Can you work these out from the drawing? Everything is in mm from the part's minimum corner. A direction names the side the tool comes from. Round coordinates to 2 decimals unless told otherwise and drop trailing zeros. Loops run counter-clockwise (first coordinate to the right, second up) from the corner with the lowest first, then second, coordinate; pieces in that order, holes last. Notation, with made-up numbers: M 63,2.5 L 95,2.5 A7 cw 95,14.5 Z; hole C -33,71.5 d10. An arc over 180 degrees is marked long. One line per question, with ' | ' between items. Start each with the question number.
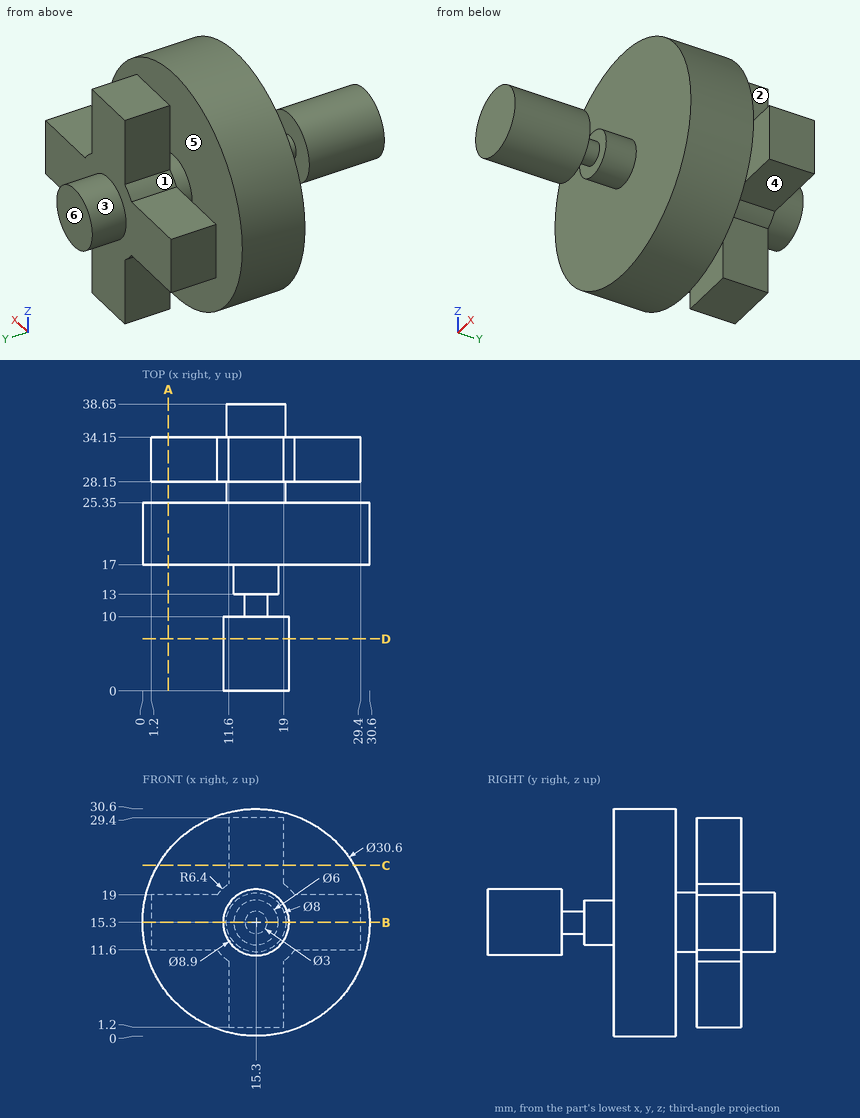
1) I'm going to push flat-ended pins straight in: pin 1 Ø6.5 at (x, y) = (4, 31) entering from +Z; pin 2 Ø8 at (y, z) = (12, 17.5) entering from +X; pin 3 Ø15.5 at (x, z) = (15.5, 8) entering from -Y; pin 4 Ø1.8 at (y, z) = (32.5, 4) entering from +X. Where does each tip first touch, or does it pass through?
2) For the marked faces 1, 2 and 3, which set-ups out of +Z, -Z, +X, -X, +Y, -Y let a thin tool reach every point of the face, with its end or its side?
3) Imagine slicing it at A-A (x = 3.5). Write out the boundary of the cut face in (y, z).
4) We'd pull the mould along Y, two halves only. Please class the marked faces 4, 5 and 6: pulls with the +Y half, pulls with the -Y half, needs draft (parallel to the pull), parting line crosses it, or undercut.
5) Imagine slicing it at B-B (z = 15.3). Write out the boundary of the cut face in (x, y), then the cut area to 3 significant figures.
6) Imagine slicing it at D-D (y = 7). Write out the boundary of the cut face in (x, z).
7) Please list where these lines run through material, in increasing order: L1, parallel to Y at x = 15.5, z = 9; L2, parallel to X at y = 32, z = 14.5; L3, parallel to Y at x = 8, z = 9.5. Write a range as from..to.
8) Imagine slicing it at C-C (z = 23). Write out the boundary of the cut face in (x, y), then the cut area to 3 significant figures.
Results are:
1) pin 1: z = 19 | pin 2: x = 19.75 | pin 3: y = 0 | pin 4: x = 19
2) face 1: +Z, -X, +Y | face 2: +Z, +X, +Y | face 3: +Y
3) outline: M 17,5.56 L 25.35,5.56 L 25.35,25.04 L 17,25.04 Z; M 28.15,11.6 L 34.15,11.6 L 34.15,19 L 28.15,19 Z
4) face 4: needs draft | face 5: undercut | face 6: pulls with the +Y half
5) outline: M 0,17 L 12.3,17 L 12.3,13 L 13.8,13 L 13.8,10 L 10.85,10 L 10.85,0 L 19.75,0 L 19.75,10 L 16.8,10 L 16.8,13 L 18.3,13 L 18.3,17 L 30.6,17 L 30.6,25.35 L 19.3,25.35 L 19.3,28.15 L 29.4,28.15 L 29.4,34.15 L 19.3,34.15 L 19.3,38.65 L 11.3,38.65 L 11.3,34.15 L 1.2,34.15 L 1.2,28.15 L 11.3,28.15 L 11.3,25.35 L 0,25.35 Z | area: 605 mm²
6) outline: C 15.3,15.3 d8.9
7) L1: 17..25.35, 28.15..34.15 | L2: 1.2..29.4 | L3: 17..25.35
8) outline: M 2.08,17 L 28.52,17 L 28.52,25.35 L 2.08,25.35 Z; M 11.6,28.15 L 19,28.15 L 19,34.15 L 11.6,34.15 Z | area: 265 mm²
